Can you work these out from the model? Positions are in its coordinate system, mm. A direction names the side the tool comes from. Give positions to 0.01 mm unless a question says otherwise; leave off trailing zeros. Order: outer loops, then holes, each group sorted by start corner. A loop starts at its lowest first (then second) coordinate and runs counter-clockwise, first axis right, second up. Notation, with made-up numbers: M -29,7 L 15,7 A13 ccw 15,25 Z; hole C -37,88 d10. An arc over 180 degrees is marked long. Use one line per item in the form item = value. Start each with the question number.
1. I need wall thicknesses on L1, parallel to Y at x = 0, z = 13.75; L2, parallel to X at y = -4.5, z = 9; L3, parallel to Y at x = -20, z = 18. Which ranges of each line are inside material? Lowest first, please.
2. I want a section at C-C, the plane z = 11.75. Count the separate pieces of the cut face and the enclosed holes in it, and give its area (3 significant figures).
3. For faces 3 (the face through (-6.76, 1.82, 11.39)), 4 (the face through (13.91, 6.82, 11.39)), which set-ups out of +Z, -Z, +X, -X, +Y, -Y let a thin tool reach every point of the face, with its end or its side?
4. Will these pins go through, and if not, where does the flat tip stop? P1, Ø2.5, axis at x = -18.5, y = -7.5, coming from the +Z side; P2, Ø4, axis at x = -4.5, y = 12, coming from the +Z side; P3, Ø5, axis at x = 0, y = 0, coming from the +Z side; P4, Ø2, axis at x = 7.5, z = 20, coming from the +Y side.
5. I want a section at A-A, the plane y = 0. List the corners of the cut face in (x, z) for me.
6. We'd pull the mould along X, two halves only. Please class faces 1 (the face through (8.636, 12.858, 11.388)), 2 (the face through (-15, -15, 3.5)): +X half, -X half, draft (parallel to the pull), parting line (faces both ways), or undercut.
```python
from build123d import *

# Parameters (mm, degrees)
SKICA1_R                 = 25.75
P_IDAT_VYSUNUT_M1_DEPTH  = 26
SKO_EPINA1_START         = 3.5
SKO_EPINA1_OUTLINE_R     = 24.25
SKO_EPINA1_DEPTH         = 22.5
SKICA2_R                 = 17
ODEBRAT_VYSUNUT_M1_DEPTH = 45.745111465
ZAOBLIT1_R               = 2
SKICA3_R                 = 4
P_IDAT_VYSUNUT_M2_DEPTH  = 16


# Read off the part's stored shape, not the designer's step: Skořepina1
with BuildPart() as part:
    # Skica1 → Přidat vysunutím1 (new body)
    with BuildSketch(Plane.XY):
        with Locations(Location((0, 0, 0), (0, 0, 180))):
            Circle(SKICA1_R)
    extrude(amount=P_IDAT_VYSUNUT_M1_DEPTH)

    # Skořepina1 outline → Skořepina1 (cut)
    with BuildSketch(Plane.XY.offset(SKO_EPINA1_START)):
        Circle(SKO_EPINA1_OUTLINE_R)
    extrude(amount=SKO_EPINA1_DEPTH, mode=Mode.SUBTRACT)

    # Skica2 → Odebrat vysunutím1 (cut, through all)
    with BuildSketch(Plane(origin=(0, 0, 0), x_dir=(-1, 0, 0), z_dir=(0, 0, -1))):
        Circle(SKICA2_R)
    extrude(amount=-ODEBRAT_VYSUNUT_M1_DEPTH, mode=Mode.SUBTRACT)

    # Zaoblit1
    zaoblit1_edges = [part.edges().sort_by_distance(p)[0] for p in [
        (25.75, 0, 0),
    ]]
    fillet(zaoblit1_edges, radius=ZAOBLIT1_R)

    # Skica3 → Přidat vysunutím2 (add)
    with BuildSketch(Plane.XY.offset(3.5)):
        with BuildLine():
            Line((-1.05, 24.227257377), (-1.05, 6.920801977))
            ThreePointArc((-1.05, 6.920801977), (-1.811733316, 6.761480784), (-2.551074314, 6.518590326))
            Line((-2.551074314, 6.518590326), (-11.204302014, 21.506420352))
            ThreePointArc((-11.204302014, 21.506420352), (-12.125, 21.001116042), (-13.022955362, 20.456420352))
            Line((-13.022955362, 20.456420352), (-4.369727662, 5.468590326))
            ThreePointArc((-4.369727662, 5.468590326), (-4.949747468, 4.949747468), (-5.468590326, 4.369727662))
            Line((-5.468590326, 4.369727662), (-20.456420352, 13.022955362))
            ThreePointArc((-20.456420352, 13.022955362), (-21.001116042, 12.125), (-21.506420352, 11.204302014))
            Line((-21.506420352, 11.204302014), (-6.518590326, 2.551074314))
            ThreePointArc((-6.518590326, 2.551074314), (-6.761480784, 1.811733316), (-6.920801977, 1.05))
            Line((-6.920801977, 1.05), (-24.227257377, 1.05))
            ThreePointArc((-24.227257377, 1.05), (-24.25, 0), (-24.227257377, -1.05))
            Line((-24.227257377, -1.05), (-6.920801977, -1.05))
            ThreePointArc((-6.920801977, -1.05), (-6.761480784, -1.811733316), (-6.518590326, -2.551074314))
            Line((-6.518590326, -2.551074314), (-21.506420352, -11.204302014))
            ThreePointArc((-21.506420352, -11.204302014), (-21.001116042, -12.125), (-20.456420352, -13.022955362))
            Line((-20.456420352, -13.022955362), (-5.468590326, -4.369727662))
            ThreePointArc((-5.468590326, -4.369727662), (-4.949747468, -4.949747468), (-4.369727662, -5.468590326))
            Line((-4.369727662, -5.468590326), (-13.022955362, -20.456420352))
            ThreePointArc((-13.022955362, -20.456420352), (-12.125, -21.001116042), (-11.204302014, -21.506420352))
            Line((-11.204302014, -21.506420352), (-2.551074314, -6.518590326))
            ThreePointArc((-2.551074314, -6.518590326), (-1.811733316, -6.761480784), (-1.05, -6.920801977))
            Line((-1.05, -6.920801977), (-1.05, -24.227257377))
            ThreePointArc((-1.05, -24.227257377), (0, -24.25), (1.05, -24.227257377))
            Line((1.05, -24.227257377), (1.05, -6.920801977))
            ThreePointArc((1.05, -6.920801977), (1.811733316, -6.761480784), (2.551074314, -6.518590326))
            Line((2.551074314, -6.518590326), (11.204302014, -21.506420352))
            ThreePointArc((11.204302014, -21.506420352), (12.125, -21.001116042), (13.022955362, -20.456420352))
            Line((13.022955362, -20.456420352), (4.369727662, -5.468590326))
            ThreePointArc((4.369727662, -5.468590326), (4.949747468, -4.949747468), (5.468590326, -4.369727662))
            Line((5.468590326, -4.369727662), (20.456420352, -13.022955362))
            ThreePointArc((20.456420352, -13.022955362), (21.001116042, -12.125), (21.506420352, -11.204302014))
            Line((21.506420352, -11.204302014), (6.518590326, -2.551074314))
            ThreePointArc((6.518590326, -2.551074314), (6.761480784, -1.811733316), (6.920801977, -1.05))
            Line((6.920801977, -1.05), (24.227257377, -1.05))
            ThreePointArc((24.227257377, -1.05), (24.25, 0), (24.227257377, 1.05))
            Line((24.227257377, 1.05), (6.920801977, 1.05))
            ThreePointArc((6.920801977, 1.05), (6.761480784, 1.811733316), (6.518590326, 2.551074314))
            Line((6.518590326, 2.551074314), (21.506420352, 11.204302014))
            ThreePointArc((21.506420352, 11.204302014), (21.001116042, 12.125), (20.456420352, 13.022955362))
            Line((20.456420352, 13.022955362), (5.468590326, 4.369727662))
            ThreePointArc((5.468590326, 4.369727662), (4.949747468, 4.949747468), (4.369727662, 5.468590326))
            Line((4.369727662, 5.468590326), (13.022955362, 20.456420352))
            ThreePointArc((13.022955362, 20.456420352), (12.125, 21.001116042), (11.204302014, 21.506420352))
            Line((11.204302014, 21.506420352), (2.551074314, 6.518590326))
            ThreePointArc((2.551074314, 6.518590326), (1.811733316, 6.761480784), (1.05, 6.920801977))
            Line((1.05, 6.920801977), (1.05, 24.227257377))
            ThreePointArc((1.05, 24.227257377), (0, 24.25), (-1.05, 24.227257377))
        make_face()
        Circle(SKICA3_R, mode=Mode.SUBTRACT)
    extrude(amount=P_IDAT_VYSUNUT_M2_DEPTH)


solid = part.part
```
Check result:
q1.L1 = -25.75 to -4, 4 to 25.75
q1.L2 = -25.35 to -23.83, -9.89 to -5.69, -5.36 to 5.36, 5.69 to 9.89, 23.83 to 25.35
q1.L3 = -16.22 to -13.71, -12.76 to -10.33, -1.05 to 1.05, 10.33 to 12.76, 13.71 to 16.22
q2.separate_pieces = 1
q2.enclosed_holes = 13
q2.area = 774 mm2
q3.face_3 = +Z, -Z
q3.face_4 = +Z
q4.P1 = 3.5
q4.P2 = 19.5
q4.P3 = through
q4.P4 = 24.92
q5.outline = M -25.75,2 A2 ccw -23.75,0 L -17,0 L -17,3.5 L -4,3.5 L -4,19.5 L -24.25,19.5 L -24.25,26 L -25.75,26 Z; M 4,3.5 L 17,3.5 L 17,0 L 23.75,0 A2 ccw 25.75,2 L 25.75,26 L 24.25,26 L 24.25,19.5 L 4,19.5 Z
q6.face_1 = undercut
q6.face_2 = undercut
